from build123d import *

# Parameters (mm, degrees)
SKETCH2_R           = 1.5875
BOSS_EXTRUDE1_DEPTH = 6.35
SKETCH3_W           = 86.520299057
SKETCH3_H           = 50.752816227
CUT_EXTRUDE1_DEPTH  = 22.86
SCALE1_SCALE        = 2
SKETCH4_W           = 272.729370393
SKETCH4_H           = 354.83187758
CUT_EXTRUDE2_DEPTH  = 5.08


with BuildPart() as part:
    # Sketch2 → Boss-Extrude1 (new body)
    # profile 1 of 3: a face of its own
    with BuildSketch(Plane.XY):
        with BuildLine():
            ThreePointArc((1.670610722, 3.717638474), (6.757246034, 4.420597856), (9.525541119, 0.095721787))
            Line((9.525541119, 0.095721787), (14.182207787, 0.095721787))
            ThreePointArc((14.182207787, 0.095721787), (17.357207787, 3.270721787), (20.532207787, 0.095721787))
            Line((20.532207787, 0.095721787), (35.983874452, 0.095721787))
            Line((35.983874452, 0.095721787), (35.983874452, 4.329055121))
            Line((35.983874452, 4.329055121), (40.217207786, 4.329055121))
            Line((40.217207786, 4.329055121), (40.217207786, 0.095721787))
            Line((40.217207786, 0.095721787), (61.383874452, 0.095721787))
            Line((61.383874452, 0.095721787), (61.383874452, 3.270721787))
            Line((61.383874452, 3.270721787), (65.617207786, 3.270721787))
            Line((65.617207786, 3.270721787), (65.617207786, 0.095721787))
            Line((65.617207786, 0.095721787), (103.86369276, 0.095721787))
            ThreePointArc((103.86369276, 0.095721787), (103.701399804, 0.51971831), (103.297478426, 0.726985228))
            add(Edge.make_bspline(
                [(103.297478426, 0.726985228), (103.278401428, 0.729063962), (102.555454876, 0.807955214), (101.062938142, 0.9797924), (98.757762781, 1.268659765), (96.264687204, 1.604159637), (93.594492647, 1.985539835), (90.758742018, 2.410830368), (87.769477293, 2.877005798), (84.639221741, 3.37990378), (81.380911453, 3.914330069), (78.007857734, 4.474123419), (74.533703974, 5.052218069), (70.972402786, 5.640770262), (67.338193058, 6.231252409), (63.64558795, 6.814592878), (59.909367026, 7.381298257), (56.144575667, 7.921621871), (52.366523305, 8.42568744), (48.590787146, 8.883665117), (44.833214748, 9.285912766), (41.109926451, 9.623146231), (37.437313832, 9.88657477), (33.832039387, 10.068065432), (30.311032911, 10.16029608), (27.586882733, 10.157568276), (26.039008587, 10.123270788), (25.632313035, 10.111855728)],
                knots=[0.036532984, 0.036532984, 0.036532984, 0.036532984, 0.036780684, 0.045920102, 0.055931764, 0.066772884, 0.07839713, 0.090754827, 0.103793165, 0.117456432, 0.131686226, 0.146421738, 0.161599998, 0.177156133, 0.193023668, 0.209134786, 0.225420633, 0.241811602, 0.258237647, 0.274628557, 0.290914287, 0.307025229, 0.322892517, 0.338448342, 0.353626207, 0.368361232, 0.373613721, 0.373613721, 0.373613721, 0.373613721], degree=3))
            add(Edge.make_bspline(
                [(25.632313035, 10.111855728), (24.937254507, 10.092346946), (23.184818676, 10.025451452), (20.426871455, 9.842671724), (17.41757594, 9.524763014), (14.581362978, 9.097201986), (11.937145196, 8.559838657), (9.777339551, 7.98685794), (8.50999095, 7.572117066), (8.045152998, 7.406999756)],
                knots=[0.373613721, 0.373613721, 0.373613721, 0.373613721, 0.382590428, 0.396252961, 0.409290412, 0.42164701, 0.433269881, 0.444109249, 0.450476502, 0.450476502, 0.450476502, 0.450476502], degree=3))
            add(Edge.make_bspline(
                [(8.045152998, 7.406999756), (7.779260681, 7.312550875), (6.851122091, 6.967807185), (5.357476635, 6.31774957), (3.688721993, 5.384292388), (2.487404704, 4.50418497), (1.86787348, 3.922488633), (1.670610722, 3.717638474)],
                knots=[0.450476502, 0.450476502, 0.450476502, 0.450476502, 0.45411864, 0.463255055, 0.471479114, 0.478755289, 0.482422896, 0.482422896, 0.482422896, 0.482422896], degree=3))
        make_face()
    # profile 2 of 3: a face of its own
    with BuildSketch(Plane.XY):
        with BuildLine():
            Line((0.000541119, 0.095721787), (9.525541119, 0.095721787))
            ThreePointArc((9.525541119, 0.095721787), (6.757246034, 4.420597856), (1.670610722, 3.717638474))
            add(Edge.make_bspline(
                [(1.670610722, 3.717638474), (1.529186884, 3.570774992), (1.119191891, 3.11301165), (0.577729932, 2.332445287), (0.184929806, 1.416285372), (0.02630969, 0.681353971), (0.000541119, 0.263637648), (0.000541119, 0.095721787)],
                knots=[0.482422896, 0.482422896, 0.482422896, 0.482422896, 0.485052318, 0.490344026, 0.494609833, 0.497833231, 0.5, 0.5, 0.5, 0.5], degree=3))
        make_face()
    # profile 3 of 3: a face of its own
    with BuildSketch(Plane.XY):
        with BuildLine():
            Line((13.380481545, 26.601119745), (8.045152998, 7.406999756))
            add(Edge.make_bspline(
                [(25.632313035, 10.111855728), (24.937254507, 10.092346946), (23.184818676, 10.025451452), (20.426871455, 9.842671724), (17.41757594, 9.524763014), (14.581362978, 9.097201986), (11.937145196, 8.559838657), (9.777339551, 7.98685794), (8.50999095, 7.572117066), (8.045152998, 7.406999756)],
                knots=[0.373613721, 0.373613721, 0.373613721, 0.373613721, 0.382590428, 0.396252961, 0.409290412, 0.42164701, 0.433269881, 0.444109249, 0.450476502, 0.450476502, 0.450476502, 0.450476502], degree=3))
            Line((25.632313035, 10.111855728), (21.351268338, 26.536748478))
            ThreePointArc((21.351268338, 26.536748478), (17.390539973, 29.623087196), (13.380481545, 26.601119745))
        make_face()
        with Locations((17.357207787, 25.495721787)):
            Circle(SKETCH2_R, mode=Mode.SUBTRACT)
    extrude(amount=BOSS_EXTRUDE1_DEPTH)

    # Sketch3 → Cut-Extrude1 (cut)
    with BuildSketch(Plane.XY.offset(6.35)):
        with Locations((79.244023981, 18.591780176)):
            Rectangle(SKETCH3_W, SKETCH3_H)
    extrude(amount=-CUT_EXTRUDE1_DEPTH, mode=Mode.SUBTRACT)


with BuildPart() as part_1:
    # Scale1: scaled about (18.859528884, 10.342075023, 3.175)
    add(part.part.scale(SCALE1_SCALE).moved(Location((-18.859528884, -10.342075023, -3.175))))

    # Sketch4 → Cut-Extrude2 (cut)
    with BuildSketch(Plane.XY.offset(9.525000538)):
        with Locations((12.859074943, 7.536544166)):
            Rectangle(SKETCH4_W, SKETCH4_H)
    extrude(amount=-CUT_EXTRUDE2_DEPTH, mode=Mode.SUBTRACT)


solid = part_1.part
Build history of the part. All positions in model axes, mm. Give positions to 0.01 mm unless a question says otherwise; leave off trailing zeros. Loops run counter-clockwise (first coordinate to the right, second up) from the corner with the lowest first, then second, coordinate; pieces in that order, holes last. Notation, with made-up numbers: (-14, -11.5) - (4, -11.5) arc R25 ccw to (4, 17.5) - close; hole circle Ø5 at (20.25, -14). An arc over 180 degrees is marked (long way). Write item = value, one per line. Start each with the question number.
1) Drop flat-ended pins along their axis: pin 1 Ø4 at (y, z) = (27, -1.5) entering from -X; pin 2 Ø5 at (x, y) = (31.5, 26.5) entering from -Z; pin 3 Ø1.5 at (y, z) = (12, 0) entering from +X; pin 4 Ø8.5 at (x, y) = (15.85, 40.65) entering from +Z (3 decimals). Give the stop position or say it passes through.
2) Pull direction X, two halves, no side cores. Call faces 1 (the cylindrical face through (16.1, 48.9, 0.6)), 2 (the cylindrical face through (15.715, -3.802, 0.582)), 3 (the flat face through (17, 13, -3.175)): +X half, -X half, draft (parallel to the pull), parting line (faces both ways), or undercut.
3) Probe probe 1 along Y at (x, z) = (45, 4.25); probe 2 along Y at (x, z) = (40, 1.5); probe 3 along X at (y, z) = (42, 4). List the from-to ranges inside material, lowest first. Write a range as from..to.
4) Band-saw the part on B-B on x = 27. Give the cut face in (y, z) (3 decimals), plus the area to 3 significant figures.
5) Band-saw the part on A-A on y = 38.5. Give the cut face in (x, z) (3 decimals).
6) Band-saw the part on C-C on y = 12. Give the cut face in (x, z) (3 decimals), plus the area to 3 significant figures.
Final values:
q1.pin_1 = 2.94
q1.pin_2 = through
q1.pin_3 = 32.05
q1.pin_4 = 4.445
q2.face_1 = parting line
q2.face_2 = undercut
q2.face_3 = draft
q3.probe_1 = -10.15..9.89
q3.probe_2 = -10.15..9.96
q3.probe_3 = 7.66..12.98, 18.73..24.03
q4.outline = (-10.151, -3.175) - (30.619, -3.175) - (30.619, 4.445) - (-10.151, 4.445) - close
q4.area = 311 mm²
q5.outline = (6.689, -3.175) - (13.518, -3.175) - (13.518, 4.445) - (6.689, 4.445) - close; (18.192, -3.175) - (24.946, -3.175) - (24.946, 4.445) - (18.192, 4.445) - close
q6.outline = (-0.677, -3.175) - (31.853, -3.175) - (31.853, 4.445) - (-0.677, 4.445) - close
q6.area = 248 mm²
